Build history of the part. All positions in model axes, mm. Round coordinates to 2 decimals unless told otherwise and drop trailing zeros. Write each loop counter-clockwise with the first axis right and the second up, starting at its lowest first coordinate (ties: lowest second). Pieces come first, ordered by that corner, then holes. Notation, with made-up numbers: (-33.5, -4) - (24.5, -4) arc R22 cw to (24.5, 31) - close; hole circle Ø11 at (30.25, -38). An arc over 180 degrees is marked (long way). Write each question's results on one line, items separated by ' | '.
from build123d import *

# Parameters (mm, degrees)
SKETCH1_R           = 4
BOSS_EXTRUDE1_DEPTH = 6
FILLET1_R           = 1


with BuildPart() as part:
    # Sketch1 → Boss-Extrude1 (new body)
    with BuildSketch(Plane(origin=(0, 0, 0), x_dir=(1, 0, 0), z_dir=(0, 1, 0))):
        Polygon((-5.135167492, 4.650812276), (-6.595305325, -2.121779363), (-1.460137834, -6.772591639), (5.135167492, -4.650812276), (6.595305325, 2.121779363), (1.460137834, 6.772591639), align=None)
        with Locations(Location((0, 0, 0), (0, 0, 270))):
            Circle(SKETCH1_R, mode=Mode.SUBTRACT)
    extrude(amount=BOSS_EXTRUDE1_DEPTH)

    # Fillet1
    fillet1_edges = [part.edges().sort_by_distance(p)[0] for p in [
        (-4.02772158, 6, 4.447185501),
        (1.837514829, 6, 5.711701958),
        (5.865236409, 6, 1.264516457),
        (0, 0, -4),
        (0, 6, -4),
        (4.02772158, 6, -4.447185501),
        (-1.837514829, 6, -5.711701958),
        (4.02772158, 0, -4.447185501),
        (5.865236409, 0, 1.264516457),
        (1.837514829, 0, 5.711701958),
        (-5.865236409, 6, -1.264516457),
        (-4.02772158, 0, 4.447185501),
        (-5.865236409, 0, -1.264516457),
        (-1.837514829, 0, -5.711701958),
    ]]
    fillet(fillet1_edges, radius=FILLET1_R - 0.0001)  # a hair under: the kernel refuses the full size


solid = part.part
(1) Slice it at A-A, the plane y = 3.75. Write the cut outline in (x, z).
Worked answers:
outline: (-6.6, 2.12) - (-5.14, -4.65) - (1.46, -6.77) - (6.6, -2.12) - (5.14, 4.65) - (-1.46, 6.77) - close; hole circle Ø8 at (0, 0)
(2) Flat gauge pins, fed straight in: pin 1 Ø3 at (y, z) = (3, 4) entering from +X; pin 2 Ø5 at (x, z) = (0, 0) entering from -Y; pin 3 Ø3 at (x, y) = (1, 4) entering from +Z; pin 4 Ø2 at (x, y) = (3, 4) entering from +Z. Where does each tip first touch, or does it go through?
Worked answers:
pin 1: stops at x = 5.6 | pin 2: passes through | pin 3: stops at z = 6.46 | pin 4: stops at z = 5.66
(3) Drill centre lines: probe 1 along X at (y, z) = (5.75, 3); probe 2 along X at (y, z) = (5.25, -2); probe 3 along Z at (x, y) = (-3, 5). Where is each one in solid material? Low to high. Write a range as [from, to].
Worked answers:
probe 1: x = [-5.12, -3.13], [3.13, 5.14] | probe 2: x = [-5.67, -3.5], [3.5, 6.54] | probe 3: z = [-5.34, -2.65], [2.65, 5.38]
(4) Two-plate mould, pull along X, no slides. Class faces 1 (the cylindrical face through (-5.597, 5.699, -1.157)), 2 (the cylindrical face through (-3.905, 2.972, -0.867)), 3 (the cylindrical face through (3.8, 0.3, -4.27)): released by +X, released by -X, zero draft, split by the parting line, or undercut.
Worked answers:
face 1: released by -X | face 2: undercut | face 3: released by +X
